Check sheet for the modelled part. Datum: model origin and axes. Units: mm. A direction names the side the tool comes from. Give positions to 0.01 mm unless a question says otherwise; leave off trailing zeros. Loops run counter-clockwise (first coordinate to the right, second up) from the corner with the lowest first, then second, coordinate; pieces in that order, holes last. Notation, with made-up numbers: (-0.5, 61.5) -> (5.5, 61.5) arc R35 cw to (5.5, 93.5) -> close; hole circle Ø1 at (72.5, 57.25). An arc over 180 degrees is marked (long way). Write each question's results on one line, items separated by ' | '. Start each with the question number.
Item 1: Cross-section at A-A on x = 0. State how many separate pieces and enclosed holes the cut face has, then the cut area to 3 significant figures.
Item 2: Cross-section at C-C on y = -3. Enter the section's corners in (x, z).
Item 3: Gauge pin test, flat ends, axial feed: pin 1 Ø12 at (x, z) = (18, 10.5) entering from -Y; pin 2 Ø22 at (x, z) = (7, -15.5) entering from +Y; pin 3 Ø1.1 at (x, z) = (-2.5, 34.5) entering from -Y. Record the tip position at first contact, or that the pin passes through.
Item 4: Access from +Z, -Z, +X, -X, +Y, -Y to the whole of each face (thin tool, end or side, straight path). Record for faces 1 (the face through (0, 12, 24)), 2 (the face through (0, 12, 35)), 3 (the face through (0.1, 8.55, 35.4)).
Item 5: Mould release check, pull along X, two halves, no side actions. Record for faces 4 (the face through (42.588, -0.563, 9.457)), 5 (the face through (0, 10, 36)), 6 (the face through (0, 13, 36)): pulls with the +X half, pulls with the -X half, needs draft (parallel to the pull), parting line crosses it, or undercut.
Item 6: Scan lines: line 1 along X through (y, z) = (9, -12); line 2 along X through (y, z) = (10.65, 0); line 3 along Y through (x, z) = (5, -39). Record each from-to range of solid material in increasing order.
from build123d import *

# Parameters (mm, degrees)
CUT_EXTRUDE_1_DEPTH = 5
EXTRUDE_START       = 6
EXTRUDE_1_DEPTH     = 6
SKETCH_8_R          = 9
CUT_EXTRUDE_2_DEPTH = 6
SKETCH_9_R          = 10
SKETCH_9_R_2        = 9
EXTRUDE_2_DEPTH     = 5


with BuildPart() as part:
    # 草图2 → 旋转1 (revolve)
    with BuildSketch(Plane.XY, mode=Mode.PRIVATE) as revolve_1_sk:
        Polygon((43.5, 0), (45.5, -9), (45.01190647, -9.108465229), (43.098914197, -0.5), (38.057271307, -0.5), (36.557271307, 11.8), (34.5, 11.8), (34.5, 8.05), (0, 8.05), (0, 8.55), (34, 8.55), (34, 12.3), (37, 12.3), (38.5, 0), align=None)
    revolve(revolve_1_sk.sketch.rotate(Axis((0, 0, 0), (0, 1, 0)), 90), axis=Axis((0, 0, 0), (0, 1, 0)))

    # 草图4 → 切除-拉伸1 (cut, symmetric)
    with BuildSketch(Plane(origin=(0, 8.55, 0), x_dir=(1, 0, 0), z_dir=(0, 1, 0))):
        with BuildLine():
            Line((-2.5, -35), (2.5, -35))
            ThreePointArc((2.5, -35), (7.5, -30), (2.5, -25))
            Line((2.5, -25), (-2.5, -25))
            ThreePointArc((-2.5, -25), (-7.5, -30), (-2.5, -35))
        make_face()
    extrude(amount=CUT_EXTRUDE_1_DEPTH, both=True, mode=Mode.SUBTRACT)

    # 草图6 → 凸台-拉伸1 (add)
    with BuildSketch(Plane(origin=(0, 8.55, 0), x_dir=(1, 0, 0), z_dir=(0, 1, 0)).offset(EXTRUDE_START)):
        with BuildLine():
            Line((-2.5, -24), (2.5, -24))
            ThreePointArc((2.5, -24), (8.5, -30), (2.5, -36))
            Line((2.5, -36), (-2.5, -36))
            ThreePointArc((-2.5, -36), (-8.5, -30), (-2.5, -24))
        make_face()
        with BuildLine():
            Line((-2.5, -25), (2.5, -25))
            ThreePointArc((2.5, -25), (7.5, -30), (2.5, -35))
            Line((2.5, -35), (-2.5, -35))
            ThreePointArc((-2.5, -35), (-7.5, -30), (-2.5, -25))
        make_face(mode=Mode.SUBTRACT)
    extrude(amount=-EXTRUDE_1_DEPTH)

    # 草图8 → 切除-拉伸2 (cut)
    with BuildSketch(Plane(origin=(0, 8.55, 0), x_dir=(1, 0, 0), z_dir=(0, 1, 0))):
        with Locations(Location((0, 5, 0), (0, 0, 270))):
            Circle(SKETCH_8_R)
    extrude(amount=-CUT_EXTRUDE_2_DEPTH, mode=Mode.SUBTRACT)

    # 草图9 → 凸台-拉伸2 (add)
    with BuildSketch(Plane.XZ.offset(-8.05)):
        with Locations(Location((0, -5, 0), (0, 0, 270))):
            Circle(SKETCH_9_R)
        with Locations(Location((0, -5, 0), (0, 0, 90))):
            Circle(SKETCH_9_R_2, mode=Mode.SUBTRACT)
    extrude(amount=EXTRUDE_2_DEPTH)


solid = part.part
Answer sheet:
1) separate pieces: 3 | enclosed holes: 0 | area: 72.6 mm²
2) outline: circle Ø88.33 at (0, 0); hole circle Ø87.31 at (0, 0)
3) pin 1: stops at y = 8.05 | pin 2: stops at y = 8.55 | pin 3: stops at y = 8.55
4) face 1: +Y | face 2: +Y, -Y | face 3: -Y
5) face 4: parting line crosses it | face 5: undercut | face 6: needs draft
6) line 1: x = -35.43 to -34.89, -32.35 to -31.81, 31.81 to 32.35, 34.89 to 35.43 | line 2: x = -37.2 to -36.7, -34.5 to -34, 34 to 34.5, 36.7 to 37.2 | line 3: y = -0.5 to 0
